Geometry: final body of the model. Coordinates: model frame, mm. A direction names the side the tool comes from. Coordinates: 2 decimals unless noted, no trailing zeros. Loops run counter-clockwise (first coordinate to the right, second up) from the corner with the lowest first, then second, coordinate; pieces in that order, holes last. Notation, with made-up numbers: (39.25, 43) - (46.25, 43) arc R27 cw to (46.25, 75) - close; hole circle Ø4 at (-37, -18). An arc over 180 degrees is marked (long way). Put each result on its own line as item: value. Start each with the question number.
1) Reachability of faces 4 (the flat face through (-14.25, 7, 150)), 5 (the flat face through (-18, 12.2, 150)) from +Z, -Z, +X, -X, +Y, -Y: full face, straight path, thin tool, end or side. Return the list, or none.
2) Material intervals for line 1 along X through (y, z) = (7.25, 86.5); line 2 along X through (y, z) = (-9.25, 52.5); line 3 along X through (y, z) = (9.75, 102), sorted ascending. Write a range as from..to.
3) Draft query along X for faces 1 (the flat face through (-21.5, -4, 150)), 2 (the flat face through (14.25, 7, 150)), 3 (the flat face through (17, 12.2, 150)). Return one class per face: +X half, -X half, draft (parallel to the pull), parting line (faces both ways), or undercut.
4) Section A-A on z = 136. Output: boundary loops of the cut face in (x, y), and give its area (3 significant figures).
5) Section B-B on x = 0.5. Output: boundary loops of the cut face in (y, z), and give its area (3 significant figures).
6) Contact query for flat-ended pins moving along their axis: pin 1 Ø1.3 at (y, z) = (5.5, 212) entering from -X; pin 2 Ø12 at (x, z) = (-5.5, 206) entering from +Y. Output: stop coordinate, or through.
```python
from build123d import *

# Parameters (mm, degrees)
SKETCH1_W           = 43
SKETCH1_H           = 24.4
BOSS_EXTRUDE1_DEPTH = 304
FILLET1_R           = 0.8
SKETCH3_W           = 3
SKETCH3_H           = 4.3
CUT_EXTRUDE1_DEPTH  = 306.00342621
SKETCH5_W           = 28.5
SKETCH5_H           = 10
CUT_EXTRUDE2_DEPTH  = 306.00342621
SKETCH6_W           = 4.2
SKETCH6_H           = 8
CUT_EXTRUDE3_DEPTH  = 306.00342621


with BuildPart() as part:
    # Sketch1 → Boss-Extrude1 (new body)
    with BuildSketch(Plane.XY):
        Rectangle(SKETCH1_W, SKETCH1_H)
    extrude(amount=BOSS_EXTRUDE1_DEPTH)

    # Fillet1
    fillet1_edges = [part.edges().sort_by_distance(p)[0] for p in [
        (21.5, -12.2, 152),
        (-21.5, -12.2, 152),
        (-21.5, 12.2, 152),
        (21.5, 12.2, 152),
    ]]
    fillet(fillet1_edges, radius=FILLET1_R)

    # Sketch3 → Cut-Extrude1 (cut, through all)
    with BuildSketch(Plane(origin=(0, 0, 0), x_dir=(-1, 0, 0), z_dir=(0, 0, -1))):
        with Locations((-20, 6.15)):
            Rectangle(SKETCH3_W, SKETCH3_H)
        with Locations((20, 6.15)):
            Rectangle(SKETCH3_W, SKETCH3_H)
    extrude(amount=-CUT_EXTRUDE1_DEPTH, mode=Mode.SUBTRACT)

    # Sketch5 → Cut-Extrude2 (cut, through all)
    with BuildSketch(Plane(origin=(0, 0, 0), x_dir=(-1, 0, 0), z_dir=(0, 0, -1))):
        with Locations((0, 7.2)):
            Rectangle(SKETCH5_W, SKETCH5_H)
    extrude(amount=-CUT_EXTRUDE2_DEPTH, mode=Mode.SUBTRACT)

    # Sketch6 → Cut-Extrude3 (cut, through all)
    with BuildSketch(Plane(origin=(0, 0, 0), x_dir=(-1, 0, 0), z_dir=(0, 0, -1))):
        with Locations((-15, -12.2)):
            Rectangle(SKETCH6_W, SKETCH6_H)
        with Locations((15, -12.2)):
            Rectangle(SKETCH6_W, SKETCH6_H)
    extrude(amount=-CUT_EXTRUDE3_DEPTH, mode=Mode.SUBTRACT)


solid = part.part
```
Answer block:
1. face 4: +Z, -Z, +Y
1. face 5: +Z, -Z, +X, -X, +Y
2. line 1: x = -18.5..-14.25, 14.25..18.5
2. line 2: x = -21.5..-17.1, -12.9..12.9, 17.1..21.5
2. line 3: x = -21.5..-14.25, 14.25..21.5
3. face 1: -X half
3. face 2: undercut
3. face 3: draft
4. outline: (-21.5, -11.4) arc R0.8 ccw to (-20.7, -12.2) - (-17.1, -12.2) - (-17.1, -8.2) - (-12.9, -8.2) - (-12.9, -12.2) - (12.9, -12.2) - (12.9, -8.2) - (17.1, -8.2) - (17.1, -12.2) - (20.7, -12.2) arc R0.8 ccw to (21.5, -11.4) - (21.5, 4) - (18.5, 4) - (18.5, 8.3) - (21.5, 8.3) - (21.5, 11.4) arc R0.8 ccw to (20.7, 12.2) - (14.25, 12.2) - (14.25, 2.2) - (-14.25, 2.2) - (-14.25, 12.2) - (-20.7, 12.2) arc R0.8 ccw to (-21.5, 11.4) - (-21.5, 8.3) - (-18.5, 8.3) - (-18.5, 4) - (-21.5, 4) - close
4. area: 704 mm²
5. outline: (-12.2, 0) - (2.2, 0) - (2.2, 304) - (-12.2, 304) - close
5. area: 4,380 mm²
6. pin 1: stops at x = -18.5
6. pin 2: stops at y = 2.2
